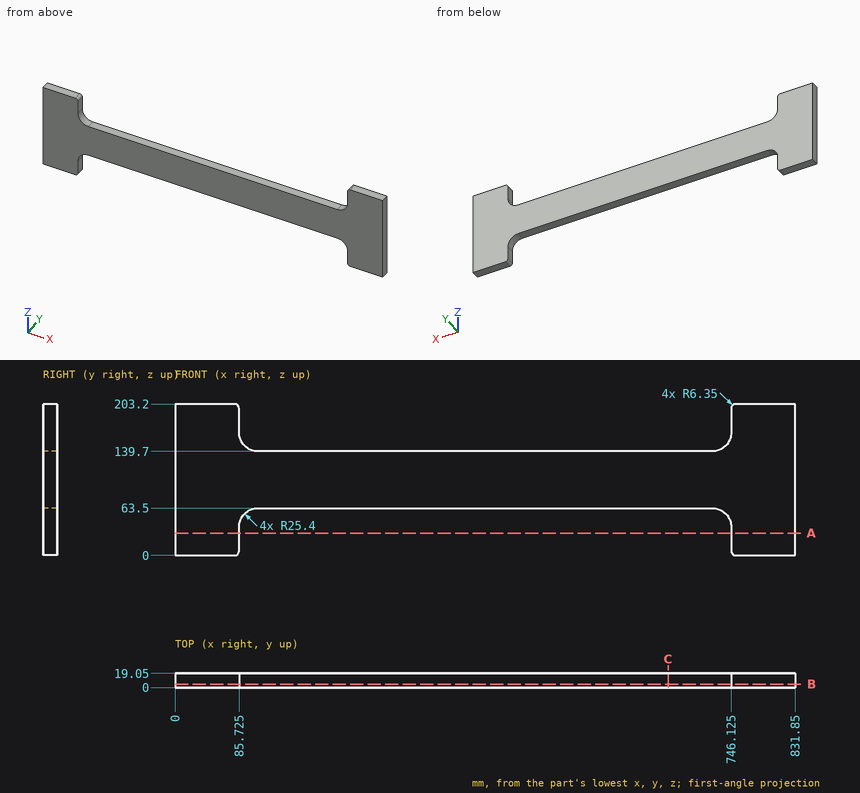
Study the drawing (mm; zero at the part's minimum x, y, z) and answer. Give positions to 0.01 mm unless a question says otherwise; leave off trailing zeros. Loops run counter-clockwise (first coordinate to the right, second up) from the corner with the lowest first, then second, coordinate; pieces in that order, holes last. Notation, with made-up numbers: M 28.25,-22.5 L 39.25,-22.5 A22 ccw 39.25,7.5 Z; hole C 87,39 d9. An arc over 180 degrees is marked long. Use CSV: the item, a comma, the result in double quotes.
1) Find section B-B on y = 4.5. Write down the section's boundary in (x, z) (3 decimals), plus the area to 3 significant figures.
Answer:
outline,"M 0,0 L 79.375,0 A6.35 ccw 85.725,6.35 L 85.725,38.1 A25.4 cw 111.125,63.5 L 720.725,63.5 A25.4 cw 746.125,38.1 L 746.125,6.35 A6.35 ccw 752.475,0 L 831.85,0 L 831.85,203.2 L 752.475,203.2 A6.35 ccw 746.125,196.85 L 746.125,165.1 A25.4 cw 720.725,139.7 L 111.125,139.7 A25.4 cw 85.725,165.1 L 85.725,196.85 A6.35 ccw 79.375,203.2 L 0,203.2 Z"
area,"85,700 mm^2"
2) Find section A-A on z = 30. Write down the section's boundary in (x, y) (3 decimals), plus the area to 3 significant figures.
Answer:
outline,"M 0,0 L 85.725,0 L 85.725,19.05 L 0,19.05 Z; M 746.125,0 L 831.85,0 L 831.85,19.05 L 746.125,19.05 Z"
area,"3,270 mm^2"
3) Find section C-C on x = 661.5. Write down the section's boundary in (y, z).
Answer:
outline,"M 0,63.5 L 19.05,63.5 L 19.05,139.7 L 0,139.7 Z"
4) Given P1, Ø1.5, axis at x = 709.5, y = 4, coming from the -Z side; P2, Ø5, axis at x = 191, y = 8, coming from the +Z side, each flat-ended and moving along its own axis, determine where each tip first touches the part or whether it passes through.
Answer:
P1,"z = 63.5"
P2,"z = 139.7"
5) Consider L1, parallel to X at y = 14.25, z = 177 (3 decimals); L2, parallel to Z at x = 169.5, y = 5.5; L3, parallel to X at y = 16.5, z = 47.5. Determine where each line is inside the solid, lowest interval first.
Answer:
L1,"0 to 85.725, 746.125 to 831.85"
L2,"63.5 to 139.7"
L3,"0 to 87.53, 744.32 to 831.85"
